For this review, use the dimensioned drawing (mm, ordinates from the lowest corner) and the shaded views. A direction names the side the tool comes from. Give positions to 0.01 mm unless a question says otherwise; leave off trailing zeros. Write each loop counter-clockwise with the first axis right and the second up, starting at its lowest first coordinate (ties: lowest second). Pieces come first, ordered by that corner, then holes.
1) We need section B-B on x = 30. Give the boundary of the cut face in (y, z).
2) For P1, Ø2, axis at y = 18, z = 36, coming from the -X side; P2, Ø5, axis at x = 47, z = 36, coming from the -Y side, all flat-tipped, find the tip position at first contact; note any pin that passes through.
3) Wall thickness on line 1 along Y through (x, z) = (35, 4); line 2 along Y through (x, z) = (39.5, 25.5); line 3 along X through (y, z) = (31.5, 29): over which ranges is each line inside the solid? List them lowest first.
4) Machinability: for the marked faces 5, 6 and 7, which of the approach directions +Z, -Z, +X, -X, +Y, -Y give a long, thin tool a straight path to every point of the face, cutting with its end or side? Answer none if there is none.
5) Draft analysis for pull direction Y (two halves, no side actions). For the marked faces 1, 2, 3 and 4, state which applies: pulls with the +Y half, pulls with the -Y half, needs draft (parallel to the pull), parting line crosses it, or undercut.
6) We need section A-A on z = 31. Give the boundary of the cut face in (x, y).
7) We need section D-D on y = 17. Give the boundary of the cut face in (x, z).
8) We need section C-C on z = 18.5. Give the boundary of the cut face in (x, y), and give its area (3 significant figures).
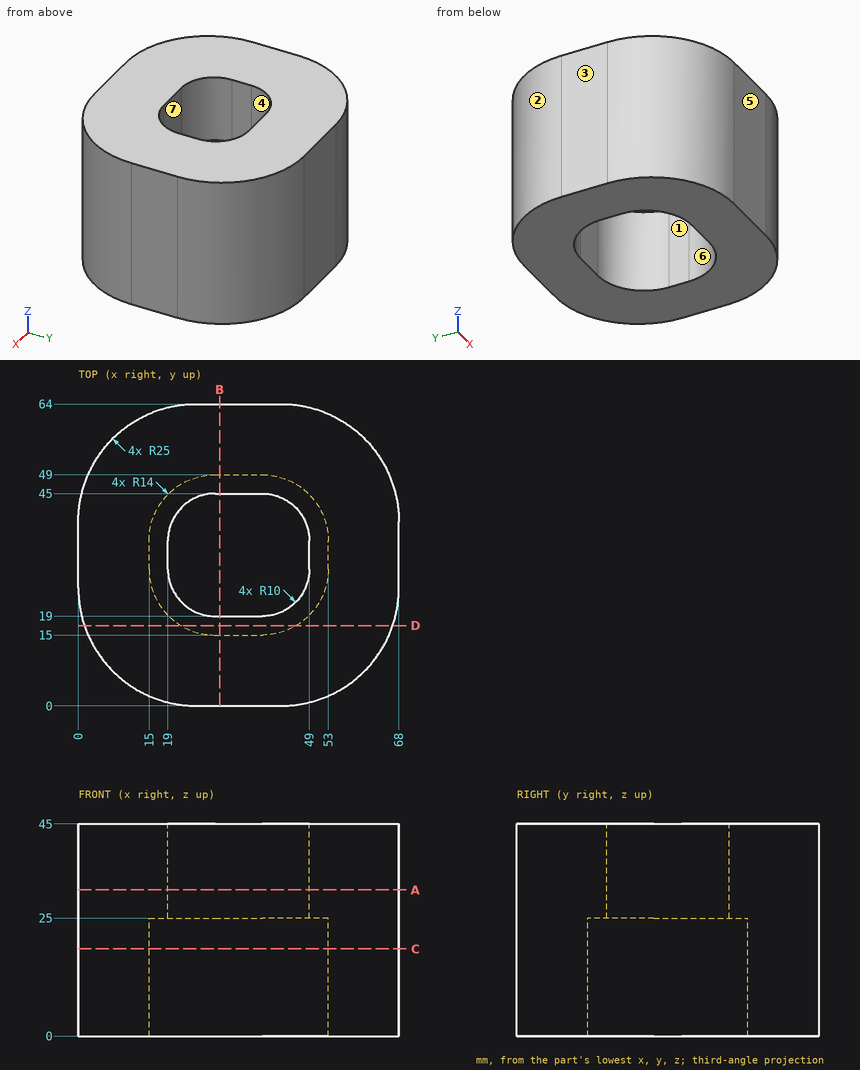
Results list:
1. outline: (0, 0) - (15, 0) - (15, 25) - (19, 25) - (19, 45) - (0, 45) - close; (45, 25) - (49, 25) - (49, 0) - (64, 0) - (64, 45) - (45, 45) - close
2. P1: stops at x = 0.73
2. P2: stops at y = 0.05
3. line 1: y = 0 to 15, 49 to 64
3. line 2: y = 0 to 19.01, 44.99 to 64
3. line 3: x = 0 to 19, 49 to 68
4. face 5: +Z, -Z, +X, -X, -Y
4. face 6: -Z
4. face 7: +Z, -Z
5. face 1: undercut
5. face 2: pulls with the +Y half
5. face 3: needs draft
5. face 4: undercut
6. outline: (0, 25) arc R25 ccw to (25, 0) - (43, 0) arc R25 ccw to (68, 25) - (68, 39) arc R25 ccw to (43, 64) - (25, 64) arc R25 ccw to (0, 39) - close; hole (19, 29) arc R10 ccw to (29, 19) - (39, 19) arc R10 ccw to (49, 29) - (49, 35) arc R10 ccw to (39, 45) - (29, 45) arc R10 ccw to (19, 35) - close
7. outline: (1.31, 0) - (21.79, 0) - (21.79, 25) - (46.21, 25) - (46.21, 0) - (66.69, 0) - (66.69, 45) - (1.31, 45) - close
8. outline: (0, 25) arc R25 ccw to (25, 0) - (43, 0) arc R25 ccw to (68, 25) - (68, 39) arc R25 ccw to (43, 64) - (25, 64) arc R25 ccw to (0, 39) - close; hole (15, 29) arc R14 ccw to (29, 15) - (39, 15) arc R14 ccw to (53, 29) - (53, 35) arc R14 ccw to (39, 49) - (29, 49) arc R14 ccw to (15, 35) - close
8. area: 2,690 mm2
